```python
from build123d import *

# Parameters (mm, degrees)
SALIENTE_EXTRUIR1_DEPTH = 2
SALIENTE_EXTRUIR3_DEPTH = 2
CROQUIS3_R              = 2
SALIENTE_EXTRUIR4_DEPTH = 5
SALIENTE_EXTRUIR5_DEPTH = 32.48


with BuildPart() as part:
    # Croquis1 → Saliente-Extruir1 (new body)
    with BuildSketch(Plane(origin=(0, 0, 0), x_dir=(1, 0, 0), z_dir=(0, 1, 0))):
        Polygon((0, 0), (0, 4), (4.242640687, 8.242640687), (19.242640687, 8.242640687), (19.242640687, 18.242640687), (29.242640687, 18.242640687), (29.242640687, 8.242640687), (59.242640687, 8.242640687), (59.242640687, 18.242640687), (69.242640687, 18.242640687), (69.242640687, 8.242640687), (84.242640687, 8.242640687), (88.485281374, 4), (88.485281374, 0), (84.242640687, -4.242640687), (69.242640687, -4.242640687), (69.242640687, -14.242640687), (59.242640687, -14.242640687), (59.242640687, -4.242640687), (29.242640687, -4.242640687), (29.242640687, -14.242640687), (19.242640687, -14.242640687), (19.242640687, -4.242640687), (4.242640687, -4.242640687), align=None)
    extrude(amount=SALIENTE_EXTRUIR1_DEPTH)

    # Croquis2 → Saliente-Extruir3 (add)
    with BuildSketch(Plane(origin=(0, 2, 0), x_dir=(1, 0, 0), z_dir=(0, 1, 0))):
        with BuildLine():
            ThreePointArc((59.242640745, 0), (57.242640745, 2), (59.242640745, 4))
            Line((59.242640745, 4), (69.242640687, 4))
            ThreePointArc((69.242640687, 4), (71.242640687, 2), (69.242640687, 0))
            Line((69.242640687, 0), (59.242640745, 0))
        make_face()
        with BuildLine():
            Line((19.242640687, 0), (29.242640687, 0))
            ThreePointArc((29.242640687, 0), (31.242640629, 2), (29.242640687, 4))
            Line((29.242640687, 4), (19.242640687, 4))
            ThreePointArc((19.242640687, 4), (17.242640687, 2), (19.242640687, 0))
        make_face()
    extrude(amount=SALIENTE_EXTRUIR3_DEPTH)

    # Croquis3 → Saliente-Extruir4 (add)
    with BuildSketch(Plane(origin=(0, 2, 0), x_dir=(1, 0, 0), z_dir=(0, 1, 0))):
        with Locations((84.242640687, 2)):
            Circle(CROQUIS3_R)
        with Locations((4.242640687, 2)):
            Circle(CROQUIS3_R)
    extrude(amount=SALIENTE_EXTRUIR4_DEPTH)

    # Croquis4 → Saliente-Extruir5 (add)
    with BuildSketch(Plane.XY.offset(14.242640687)):
        with BuildLine():
            Line((19.242640687, 0), (29.242640687, 0))
            ThreePointArc((29.242640687, 0), (24.242640687, -5), (19.242640687, 0))
        make_face()
        with BuildLine():
            Line((59.242640687, 0), (69.242640687, 0))
            ThreePointArc((69.242640687, 0), (64.242640687, -5), (59.242640687, 0))
        make_face()
    extrude(amount=-SALIENTE_EXTRUIR5_DEPTH)


solid = part.part
```
Geometry: final body of the model. Coordinates: model frame, mm. A direction names the side the tool comes from. Give positions to 0.01 mm unless a question says otherwise; leave off trailing zeros. Order: outer loops, then holes, each group sorted by start corner. A loop starts at its lowest first (then second) coordinate and runs counter-clockwise, first axis right, second up. Notation, with made-up numbers: (47, 6) -> (101, 6) arc R21 ccw to (101, 32) -> close; hole circle Ø3 at (30, -0.5). An arc over 180 degrees is marked (long way). Write each question's results on one line, items separated by ' | '. Start each with the question number.
1) First-contact query: pin 1 (4.5 mm diameter, centred on x = 21, z = -2.5, fed in from +Y); pin 2 (10 mm diameter, centred on x = 75, z = -2.5, fed in from -Y); pin 3 (0.6 mm diameter, centred on y = 1, z = 8, fed in from +X). Flat tips, straight axial feed; report the tip coordinate or a pass-through.
2) Section B-B (y = -3.5). Return loops of the section in (x, z).
3) Line query: line 1 (X direction, y = 2.5, z = -1.5); line 2 (X direction, y = 1, z = -9); line 3 (Z direction, x = 60, y = -1.5). Output: solid intervals per line, ascending. Write a range as from..to.
4) Section A-A (z = -12). Return loops of the section in (x, y).
5) Set-up query: faces 5 (the flat face through (77, 1, 4.243)), 6 (the flat face through (10, 0, -2)), 7 (the flat face through (24, 3, 0)), 8 (the flat face through (44, 0, -2)). Return all of +Z, -Z, +X, -X, +Y, -Y with unobstructed straight access to the full face (end or side cutting, diameter ignored); none if empty.
6) Section C-C (z = -2). Return loops of the section in (x, y).
7) Draft query along X for faces 1 (the flat face through (29.243, 1, -13)), 2 (the flat face through (24, 4, -2)), 3 (the flat face through (2, 1, 2)), 4 (the flat face through (12, 1, -8.243)). Return one class per face: pulls with the +X half, pulls with the -X half, needs draft (parallel to the pull), parting line crosses it, or undercut.
Calculated:
1) pin 1: y = 4 | pin 2: y = 0 | pin 3: x = 69.24
2) outline: (20.67, -18.24) -> (27.81, -18.24) -> (27.81, 14.24) -> (20.67, 14.24) -> close; (60.67, -18.24) -> (67.81, -18.24) -> (67.81, 14.24) -> (60.67, 14.24) -> close
3) line 1: 2.31..6.18, 17.31..31.18, 57.31..71.18, 82.31..86.18 | line 2: 19.24..29.24, 59.24..69.24 | line 3: -18.24..14.24
4) outline: (19.24, 0) arc R5 ccw to (29.24, 0) -> (29.24, 2) -> (19.24, 2) -> close; (59.24, 0) arc R5 ccw to (69.24, 0) -> (69.24, 2) -> (59.24, 2) -> close
5) face 5: +Z, +X, +Y, -Y | face 6: +Z, -Z, -X, -Y | face 7: +Z, +X, -X, +Y | face 8: +Z, -Z, -Y
6) outline: (0, 0) -> (19.24, 0) arc R5 ccw to (29.24, 0) -> (59.24, 0) arc R5 ccw to (69.24, 0) -> (88.49, 0) -> (88.49, 2) -> (86.24, 2) -> (86.24, 7) -> (82.24, 7) -> (82.24, 2) -> (71.24, 2) -> (71.24, 4) -> (57.24, 4) -> (57.24, 2) -> (31.24, 2) -> (31.24, 4) -> (17.24, 4) -> (17.24, 2) -> (6.24, 2) -> (6.24, 7) -> (2.24, 7) -> (2.24, 2) -> (0, 2) -> close
7) face 1: undercut | face 2: undercut | face 3: pulls with the -X half | face 4: needs draft
